Verification items for the finished model (mm, model axes). A direction names the side the tool comes from. Coordinates: 2 decimals unless noted, no trailing zeros. Order: outer loops, then holes, each group sorted by start corner. A loop starts at its lowest first (then second) coordinate and runs counter-clockwise, first axis right, second up. Notation, with made-up numbers: M 19,-16 L 35,-16 A4 cw 35,-9 Z; hole C -17,-14.75 d3. An arc over 180 degrees is marked long. Return JSON: item names as keys, results as strings. Group by question number.
Q1. Access from +Z, -Z, +X, -X, +Y, -Y to the whole of each face (thin tool, end or side, straight path). Record for faces 1 (the face through (0, 2, -4)), 2 (the face through (0, 4, -3)).
Q2. Section check A-A, the plane x = 0. Enter the section's corners in (y, z).
Q3. Section check B-B, the plane y = 2.25. Enter the section's corners in (x, z), then the cut area to 3 significant figures.
Q4. Thickness scan on probe 1 along Y at (x, z) = (1.75, 3); probe 2 along X at (y, z) = (22.5, -1.5); probe 3 along Z at (x, y) = (-2.5, 1.75). Record the ranges inside material, lowest first.
Q5. Go/stop test with flat-tipped pins: pin 1 Ø3 at (y, z) = (10.5, 1.5) entering from +X; pin 2 Ø3 at (x, z) = (3.5, -2.5) entering from +Y; pin 3 Ø4 at (x, y) = (-1.5, 7.5) entering from +Z. Record where each tip stops, or that it passes through.
Q6. Section check C-C, the plane y = 7.5. Enter the section's corners in (x, z), then the cut area to 3 significant figures.
from build123d import *

# Parameters (mm, degrees)
BOSS_EXTRUDE1_DEPTH = 4
SKETCH2_R           = 2.5
BOSS_EXTRUDE2_DEPTH = 20
FILLET1_R           = 0.2
CHAMFER1_SIZE       = 0.5


with BuildPart() as part:
    # Sketch1 → Boss-Extrude1 (new body)
    with BuildSketch(Plane(origin=(0, 0, 0), x_dir=(1, 0, 0), z_dir=(0, 1, 0))):
        Polygon((4.618802154, 0), (2.309401077, 4), (-2.309401077, 4), (-4.618802154, 0), (-2.309401077, -4), (2.309401077, -4), align=None)
    extrude(amount=BOSS_EXTRUDE1_DEPTH)

    # Sketch2 → Boss-Extrude2 (add)
    with BuildSketch(Plane(origin=(0, 4, 0), x_dir=(1, 0, 0), z_dir=(0, 1, 0))):
        with Locations(Location((0, 0, 0), (0, 0, 270))):
            Circle(SKETCH2_R)
    extrude(amount=BOSS_EXTRUDE2_DEPTH)

    # Sketch3 → Cut-Revolve1 (revolve, cut)
    with BuildSketch(Plane.XY):
        Polygon((-4.618802154, 0.7), (-3.918802154, 0), (-4.618802154, 0), align=None)
    revolve(axis=Axis((0, -1000, 0), (0, 1, 0)), mode=Mode.SUBTRACT)

    # Fillet1
    fillet1_edges = [part.edges().sort_by_distance(p)[0] for p in [
        (0, 4, -2.5),
    ]]
    fillet(fillet1_edges, radius=FILLET1_R)

    # Chamfer1
    chamfer1_edges = [part.edges().sort_by_distance(p)[0] for p in [
        (0, 24, -2.5),
    ]]
    chamfer(chamfer1_edges, length=CHAMFER1_SIZE)


solid = part.part
Numbers:
{
 "1": {"face 1": "-Z, +X, -X, +Y, -Y", "face 2": "+Y"},
 "2": {"outline": "M 0,-3.92 L 0.08,-4 L 4,-4 L 4,-2.7 A0.2 cw 4.2,-2.5 L 23.5,-2.5 L 24,-2 L 24,2 L 23.5,2.5 L 4.2,2.5 A0.2 cw 4,2.7 L 4,4 L 0.08,4 L 0,3.92 Z"},
 "3": {"outline": "M -4.62,0 L -2.31,-4 L 2.31,-4 L 4.62,0 L 2.31,4 L -2.31,4 Z", "area": "55.4 mm2"},
 "4": {"probe 1": "y = 0 to 4", "probe 2": "x = -2 to 2", "probe 3": "z = -3.67 to 3.67"},
 "5": {"pin 1": "stops at x = 2.5", "pin 2": "stops at y = 4", "pin 3": "stops at z = 2.5"},
 "6": {"outline": "C 0,0 d5", "area": "19.6 mm2"}
}
